```python
from build123d import *

# Parameters (mm, degrees)
F1_DEPTH = 25.4
F3_T     = -2.54


with BuildPart() as f1:
    # F0 (on Front) → F1 (new body)
    with BuildSketch(Plane.XZ):
        Polygon((-24.2911779621, 13.655773364), (-24.3787635118, 13.655773364), (-24.3787635118, -55.814538151), (27.4948440492, -55.814538151), (27.4948440492, 13.655773364), (27.4072584995, 13.655773364), align=None)
        with BuildLine():
            ThreePointArc((27.4072584995, 13.655773364), (1.5580402687, 39.5049915948), (-24.2911779621, 13.655773364))
            Line((-24.2911779621, 13.655773364), (27.4072584995, 13.655773364))
        make_face()
    extrude(amount=F1_DEPTH)

    # F3
    f3_openings = [f1.faces().sort_by_distance(p)[0] for p in [
        (1.55804, -25.4, -10.770056),
    ]]
    offset(amount=F3_T, openings=f3_openings, kind=Kind.INTERSECTION)

    # F4: F1 across face


with BuildPart() as f1_1:
    add(f1.part)
    add(f1.part.mirror(Plane(origin=(1.5580402687, -12.7, -55.814538151), x_dir=(1, 0, 0), z_dir=(0, 0, -1))))


solid = f1_1.part
```
Here's how the part is built. I have some questions about the finished solid (model axes, mm). A direction names the side the tool comes from. Round coordinates to 2 decimals unless told otherwise and drop trailing zeros. Order: outer loops, then holes, each group sorted by start corner. A loop starts at its lowest first (then second) coordinate and runs counter-clockwise, first axis right, second up. Notation, with made-up numbers: M -27,-7.5 L 24,-7.5 A18 ccw 24,24.5 Z; hole C 33,79 d2. An arc over 180 degrees is marked long. One line per question, with ' | ' between items.
1) For pin 1 Ø3 at (x, y) = (16, -15.5) entering from -Z; pin 2 Ø4 at (x, z) = (5.5, 17) entering from -Y; pin 3 Ø5 at (x, y) = (-2.5, -7.5) entering from -Z, each with a flat end and sliding along its axis, tell me the tip position at first contact or that it passes through.
Working result:
pin 1: z = -147.66 | pin 2: y = -2.54 | pin 3: z = -151.09
2) I want a section at A-A, the plane y = -13.25. Write out the boundary of the cut face in (x, z).
Working result:
outline: M -24.38,-125.28 L -24.29,-125.28 A25.85 ccw 27.41,-125.28 L 27.49,-125.28 L 27.49,13.66 L 27.41,13.66 A25.85 ccw -24.29,13.66 L -24.38,13.66 Z; hole M -21.84,-122.74 L -21.61,-122.74 A23.31 ccw long 24.73,-122.74 L 24.95,-122.74 L 24.95,-58.35 L -21.84,-58.35 Z; hole M -21.84,-53.27 L 24.95,-53.27 L 24.95,11.12 L 24.73,11.12 A23.31 ccw long -21.61,11.12 L -21.84,11.12 Z
3) If we mould it in two halves opening along X, with no side actions, what happens to faces 1 (the face through (1, -14, -53.275)), 2 (the face through (-21.839, -14, -21)), 3 (the face through (2.1, -12.5, 39.5)), 4 (the face through (-24.379, -13, -57))? For each: +X half, -X half, draft (parallel to the pull), parting line (faces both ways), or undercut.
Working result:
face 1: undercut | face 2: undercut | face 3: parting line | face 4: -X half
4) For faces 5 (the face through (2.106, -13.81, -148.588)), 6 (the face through (2.126, -12.522, -151.128)), which set-ups out of +Z, -Z, +X, -X, +Y, -Y let a thin tool reach every point of the face, with its end or its side?
Working result:
face 5: -Y | face 6: -Z, +Y, -Y
5) I want a section at C-C, the plane x = 3. Write out the boundary of the cut face in (y, z), then the cut area to 3 significant figures.
Working result:
outline: M -25.4,-151.09 L 0,-151.09 L 0,39.46 L -25.4,39.46 L -25.4,36.92 L -2.54,36.92 L -2.54,-53.27 L -25.4,-53.27 L -25.4,-58.35 L -2.54,-58.35 L -2.54,-148.55 L -25.4,-148.55 Z | area: 716 mm²
6) I need wall thicknesses on line 1 along Z through (x, y) = (2, -11); line 2 along X through (y, z) = (-9.5, -7); line 3 along Z through (x, y) = (-19, -16.25). Which ranges of each line are inside material? Lowest first, please.
Working result:
line 1: -151.13 to -148.59, -58.35 to -53.27, 36.96 to 39.5 | line 2: -24.38 to -21.84, 24.95 to 27.49 | line 3: -140.95 to -136.27, -58.35 to -53.27, 24.64 to 29.33
7) I want a section at B-B, the plane z = -102. Write out the boundary of the cut face in (x, y), then the cut area to 3 significant figures.
Working result:
outline: M -24.38,-25.4 L -21.84,-25.4 L -21.84,-2.54 L 24.95,-2.54 L 24.95,-25.4 L 27.49,-25.4 L 27.49,0 L -24.38,0 Z | area: 248 mm²
8) I want a section at D-D, the plane x = -17. Write out the boundary of the cut face in (y, z), then the cut area to 3 significant figures.
Working result:
outline: M -25.4,-143.28 L 0,-143.28 L 0,31.65 L -25.4,31.65 L -25.4,27.76 L -2.54,27.76 L -2.54,-53.27 L -25.4,-53.27 L -25.4,-58.35 L -2.54,-58.35 L -2.54,-139.39 L -25.4,-139.39 Z | area: 738 mm²
